from build123d import *

# Parameters (mm, degrees)
SKETCH1_R           = 27.78125
SKETCH1_R_2         = 14.29
BOSS_EXTRUDE1_DEPTH = 15.875
CUT_EXTRUDE1_DEPTH  = 16.875


with BuildPart() as part:
    # Sketch1 → Boss-Extrude1 (new body)
    with BuildSketch(Plane.XY):
        Circle(SKETCH1_R)
        Circle(SKETCH1_R_2, mode=Mode.SUBTRACT)
    extrude(amount=BOSS_EXTRUDE1_DEPTH)

    # Sketch3 → Cut-Extrude1 (cut, through all)
    with BuildSketch(Plane.XY.offset(15.875)):
        with BuildLine():
            Line((18.814306165, -16.462742285), (4.849999952, -8.400446334))
            Line((4.849999952, -8.400446334), (4.849999952, -24.525038236))
            ThreePointArc((4.849999952, -24.525038236), (-4.9e-08, -25), (-4.850000048, -24.525038217))
            Line((-4.850000048, -24.525038217), (-4.850000048, -8.4004465))
            Line((-4.850000048, -8.4004465), (-18.814306101, -16.462742358))
            ThreePointArc((-18.814306101, -16.462742358), (-21.65063507, -12.500000042), (-23.664306117, -8.062295951))
            Line((-23.664306117, -8.062295951), (-9.699999904, 0))
            Line((-9.699999904, 0), (-23.664306117, 8.062295951))
            ThreePointArc((-23.664306117, 8.062295951), (-21.65063507, 12.500000042), (-18.814306101, 16.462742358))
            Line((-18.814306101, 16.462742358), (-4.850000048, 8.4004465))
            Line((-4.850000048, 8.4004465), (-4.850000048, 24.525038217))
            ThreePointArc((-4.850000048, 24.525038217), (-4.9e-08, 25), (4.849999952, 24.525038236))
            Line((4.849999952, 24.525038236), (4.849999952, 8.400446334))
            Line((4.849999952, 8.400446334), (18.814306165, 16.462742285))
            ThreePointArc((18.814306165, 16.462742285), (21.650635119, 12.499999958), (23.664306149, 8.062295858))
            Line((23.664306149, 8.062295858), (9.700000096, 0))
            Line((9.700000096, 0), (23.664306149, -8.062295858))
            ThreePointArc((23.664306149, -8.062295858), (21.650635119, -12.499999958), (18.814306165, -16.462742285))
        make_face()
    extrude(amount=-CUT_EXTRUDE1_DEPTH, mode=Mode.SUBTRACT)


solid = part.part
Model file for the job. Use its own axes, mm. Give positions to 0.01 mm unless a question says otherwise; leave off trailing zeros. Loops run counter-clockwise (first coordinate to the right, second up) from the corner with the lowest first, then second, coordinate; pieces in that order, holes last. Notation, with made-up numbers: (50, -19.75) - (56, -19.75) arc R16 ccw to (56, -12.75) - close; hole circle Ø3 at (-0.75, -33.5). An arc over 180 degrees is marked (long way). Use one line per item in the form item = value.
(1) Cut at D-D (x = -15). Give the cut face in (y, z) (3 decimals), then the cut area to 3 significant figures.
Determined:
outline = (-23.384, 0) - (-14.261, 0) - (-14.261, 15.875) - (-23.384, 15.875) - close; (-3.06, 0) - (3.06, 0) - (3.06, 15.875) - (-3.06, 15.875) - close; (14.261, 0) - (23.384, 0) - (23.384, 15.875) - (14.261, 15.875) - close
area = 387 mm^2
(2) Drill centre lines: L1, parallel to Y at x = -19, z = 4; L2, parallel to Y at x = 15, z = 5; L3, parallel to Y at x = -9.5, z = 14. Where is each one in solid material? Low to high.
Determined:
L1 = -20.27 to -16.25, -5.37 to 5.37, 16.25 to 20.27
L2 = -23.38 to -14.26, -3.06 to 3.06, 14.26 to 23.38
L3 = -26.11 to -11.09, 11.09 to 26.11
(3) Cut at C-C (x = 0). Give the cut face in (y, z) (3 decimals).
Determined:
outline = (-27.781, 0) - (-25, 0) - (-25, 15.875) - (-27.781, 15.875) - close; (25, 0) - (27.781, 0) - (27.781, 15.875) - (25, 15.875) - close
(4) Cut at A-A (y = 0). Give the cut face in (x, z) (3 decimals).
Determined:
outline = (-27.781, 0) - (-14.29, 0) - (-14.29, 15.875) - (-27.781, 15.875) - close; (14.29, 0) - (27.781, 0) - (27.781, 15.875) - (14.29, 15.875) - close
(5) Pull direction X, two halves, no side cores. Call faces 1 (the face through (-7, 13, 15.875)), 2 (the face through (-3.617, 27.545, 7.826)), 3 (the face through (18.93, 5.33, 8.05)): pulls with the +X half, pulls with the -X half, needs draft (parallel to the pull), parting line crosses it, or undercut.
Determined:
face_1 = needs draft
face_2 = parting line crosses it
face_3 = undercut
(6) Cut at B-B (z = 10). Give the cut face in (x, y).
Determined:
outline = circle Ø55.56 at (0, 0); hole (-23.66, -8.06) arc R25 ccw to (-18.81, -16.46) - (-9.22, -10.92) arc R14.29 ccw to (-4.85, -13.44) - (-4.85, -24.53) arc R25 ccw to (4.85, -24.53) - (4.85, -13.44) arc R14.29 ccw to (9.22, -10.92) - (18.81, -16.46) arc R25 ccw to (23.66, -8.06) - (14.07, -2.52) arc R14.29 ccw to (14.07, 2.52) - (23.66, 8.06) arc R25 ccw to (18.81, 16.46) - (9.22, 10.92) arc R14.29 ccw to (4.85, 13.44) - (4.85, 24.53) arc R25 ccw to (-4.85, 24.53) - (-4.85, 13.44) arc R14.29 ccw to (-9.22, 10.92) - (-18.81, 16.46) arc R25 ccw to (-23.66, 8.06) - (-14.07, 2.52) arc R14.29 ccw to (-14.07, -2.52) - close
(7) Drop flat-ended pins along their axis: P1, Ø6, axis at x = -15, z = 12, coming from the -Y side; P2, Ø9, axis at y = -21.5, z = 5.5, coming from the -X side; P3, Ø9, axis at y = 17.5, z = 7, coming from the +X side; P4, Ø1.5, axis at x = 20.5, y = 12.5, coming from the -Z side. Give the stop position or say it passes through.
Determined:
P1 = -25.06
P2 = -21.97
P3 = 24.55
P4 = through
